For this review, take the finished solid that the model builds, in its own axes (mm). A direction names the side the tool comes from. Give positions to 0.01 mm unless a question says otherwise; leave off trailing zeros. Write each loop counter-clockwise with the first axis right and the second up, starting at its lowest first coordinate (ties: lowest second). Pieces come first, ordered by that corner, then holes.
1) We need section A-A on z = 5. Give the number of separate pieces and of enclosed holes in the cut face, and give its area (3 significant figures).
2) Machinability: for faces 5 (the face through (40, 0, 5)), 6 (the face through (58, 15, 5)), which of the approach directions +Z, -Z, +X, -X, +Y, -Y give a long, thin tool a straight path to every point of the face, cutting with its end or side? Answer none if there is none.
3) We need section C-C on x = 12. Give the boundary of the cut face in (y, z).
4) Wall thickness on line 1 along Y through (x, z) = (62, 5); line 2 along Y through (x, z) = (10, 7.5); line 3 along X through (y, z) = (11.25, 5): over which ranges is each line inside the solid? List them lowest first.
5) For P1, Ø3, axis at y = 6, z = 7.5, coming from the -X side; P2, Ø2.5, axis at y = 5, z = 5, coming from the -X side; P3, Ø2, axis at y = 5, z = 3, coming from the -X side, all flat-tipped, find the tip position at first contact; note any pin that passes through.
6) We need section B-B on y = 8. Give the boundary of the cut face in (x, z).
7) Draft analysis for pull direction Z (two halves, no side actions). For faces 1 (the face through (58, 5, 5)), 2 (the face through (2.85, 3.01, 5.07)), 3 (the face through (64.902, 7.082, 4.727)), 4 (the face through (35, 10, 10)), state which applies: pulls with the +Z half, pulls with the -Z half, needs draft (parallel to the pull), parting line crosses it, or undercut.
from build123d import *

# Parameters (mm, degrees)
ESQUISSE1_W               = 72
ESQUISSE1_H               = 20
ESQUISSE1_R               = 4
BOSS_EXTRU_1_DEPTH        = 10
CONG_1_R                  = 10
TROU_TARAUD_M5X0_82_D     = 4.2
TROU_TARAUD_M5X0_82_DEPTH = 14
CONG_2_R                  = 1


with BuildPart() as part:
    # Esquisse1 → Boss.-Extru.1 (new body)
    with BuildSketch(Plane.XY):
        with Locations((36, 10)):
            Rectangle(ESQUISSE1_W, ESQUISSE1_H)
        with Locations((10, 10)):
            Circle(ESQUISSE1_R, mode=Mode.SUBTRACT)
        with Locations((54, 10)):
            Circle(ESQUISSE1_R, mode=Mode.SUBTRACT)
    extrude(amount=BOSS_EXTRU_1_DEPTH)

    # Congé1
    cong_1_edges = [part.edges().sort_by_distance(p)[0] for p in [
        (0, 0, 5),
        (0, 20, 5),
    ]]
    fillet(cong_1_edges, radius=CONG_1_R - 0.0001)  # a hair under: the kernel refuses the full size

    # Trou taraudé M5x0.82
    with Locations(Plane(origin=(72, 0, 0), x_dir=(0, 0, -1), z_dir=(1, 0, 0))):
        with Locations((-5, 15), (-5, 5)):
            Hole(TROU_TARAUD_M5X0_82_D / 2, depth=TROU_TARAUD_M5X0_82_DEPTH)

    # Congé2
    cong_2_edges = [part.edges().sort_by_distance(p)[0] for p in [
        (72, 0, 5),
        (72, 20, 5),
    ]]
    fillet(cong_2_edges, radius=CONG_2_R)


solid = part.part
Results list:
1. separate pieces: 1
1. enclosed holes: 2
1. area: 1,180 mm2
2. face 5: +Z, -Z, +X, -X, -Y
2. face 6: +X
3. outline: (0, 0) - (6.54, 0) - (6.54, 10) - (0, 10) - close; (13.46, 0) - (20, 0) - (20, 10) - (13.46, 10) - close
4. line 1: y = 0 to 2.9, 7.1 to 12.9, 17.1 to 20
4. line 2: y = 0 to 6, 14 to 20
4. line 3: x = 0.08 to 6.2, 13.8 to 50.2, 57.8 to 72
5. P1: stops at x = 0.32
5. P2: stops at x = 0.73
5. P3: stops at x = 0.83
6. outline: (0.2, 0) - (6.54, 0) - (6.54, 10) - (0.2, 10) - close; (13.46, 0) - (50.54, 0) - (50.54, 10) - (13.46, 10) - close; (57.46, 0) - (72, 0) - (72, 10) - (57.46, 10) - close
7. face 1: undercut
7. face 2: needs draft
7. face 3: undercut
7. face 4: pulls with the +Z half
